```python
from build123d import *

# Parameters (mm, degrees)
SKETCH1_W           = 80
SKETCH1_H           = 20
BOSS_EXTRUDE1_DEPTH = 30
SKETCH2_W           = 80
SKETCH2_H           = 7
CUT_EXTRUDE1_DEPTH  = 22
SKETCH3_W           = 40
SKETCH3_H           = 20
BOSS_EXTRUDE2_DEPTH = 20
SKETCH4_R           = 2.25
CUT_EXTRUDE2_DEPTH  = 81.622577483
FILLET1_R           = 10
FILLET2_R           = 4


with BuildPart() as part:
    # Sketch1 → Boss-Extrude1 (new body)
    with BuildSketch(Plane(origin=(0, 0, 0), x_dir=(1, 0, 0), z_dir=(0, 1, 0))):
        with Locations((40, -10)):
            Rectangle(SKETCH1_W, SKETCH1_H)
    extrude(amount=BOSS_EXTRUDE1_DEPTH)

    # Sketch2 → Cut-Extrude1 (cut)
    with BuildSketch(Plane(origin=(0, 0, 0), x_dir=(-1, 0, 0), z_dir=(0, -1, 0))):
        with Locations((-40, -10)):
            Rectangle(SKETCH2_W, SKETCH2_H)
    extrude(amount=-CUT_EXTRUDE1_DEPTH, mode=Mode.SUBTRACT)

    # Sketch3 → Boss-Extrude2 (add)
    with BuildSketch(Plane(origin=(0, 30, 0), x_dir=(1, 0, 0), z_dir=(0, 1, 0))):
        with Locations((40, -10)):
            Rectangle(SKETCH3_W, SKETCH3_H)
    extrude(amount=BOSS_EXTRUDE2_DEPTH)

    # Sketch4 → Cut-Extrude2 (cut, through all)
    with BuildSketch(Plane.ZY.offset(-20)):
        with Locations((10, 40)):
            Circle(SKETCH4_R)
    extrude(amount=-CUT_EXTRUDE2_DEPTH, mode=Mode.SUBTRACT)

    # Fillet1
    fillet1_edges = [part.edges().sort_by_distance(p)[0] for p in [
        (40, 50, 0),
        (40, 50, 20),
    ]]
    fillet(fillet1_edges, radius=FILLET1_R - 0.0001)  # a hair under: the kernel refuses the full size

    # Fillet2
    fillet2_edges = [part.edges().sort_by_distance(p)[0] for p in [
        (40, 0, 0),
        (40, 0, 20),
    ]]
    fillet(fillet2_edges, radius=FILLET2_R)


solid = part.part
```
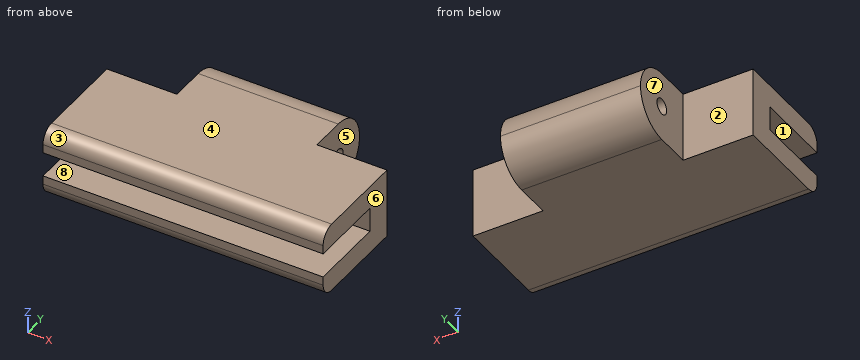
Can you work these out from the model? Positions are in its coordinate system, mm. Face numbers are marked on the shaded views. A direction names the side the tool comes from. Coordinates: 2 decimals unless noted, no trailing zeros. Loops run counter-clockwise (first coordinate to the right, second up) from the corner with the lowest first, then second, coordinate; pieces in that order, holes last. Notation, with made-up numbers: (37.5, -5) -> (62.5, -5) arc R32 ccw to (62.5, 24) -> close; hole circle Ø9 at (89.25, -40). An arc over 180 degrees is marked (long way). Answer as a JSON object with one key per item and string values.
1) Imagine slicing it at A-A (y = 17). Please give me the cut outline in (x, z).
Results:
{"outline": "(0, 0) -> (80, 0) -> (80, 6.5) -> (0, 6.5) -> close; (0, 13.5) -> (80, 13.5) -> (80, 20) -> (0, 20) -> close"}
2) Imagine slicing it at D-D (x = 17). Please give me the cut outline in (y, z), then the cut area to 3 significant figures.
Results:
{"outline": "(0, 4) arc R4 ccw to (4, 0) -> (30, 0) -> (30, 20) -> (4, 20) arc R4 ccw to (0, 16) -> (0, 13.5) -> (22, 13.5) -> (22, 6.5) -> (0, 6.5) -> close", "area": "439 mm^2"}
3) For the marked faces 4, 5, 6, 7 and 8, which set-ups out of +Z, -Z, +X, -X, +Y, -Y let a thin tool reach every point of the face, with its end or its side?
Results:
{"face 4": "+Z, +X, -X, +Y, -Y", "face 5": "+Z, -Z, +X, +Y", "face 6": "+Z, -Z, +X, +Y, -Y", "face 7": "+Z, -Z, -X, +Y", "face 8": "+X, -X, -Y"}
4) Thinking about a two-plate mould opening in Z: for the marked faces 1, 2 and 3, which applies, pulls with the +Z half, pulls with the -Z half, needs draft (parallel to the pull), parting line crosses it, or undercut?
Results:
{"face 1": "undercut", "face 2": "needs draft", "face 3": "pulls with the +Z half"}
5) For P1, Ø6, axis at x = 71.5, z = 3.5, coming from the +Y side; P2, Ø1, axis at x = 65.5, z = 11.5, coming from the -Y side; P3, Ø6, axis at y = 41.5, z = 8, coming from the -X side, each with a flat end and sliding along its axis, tell me the tip position at first contact or that it passes through.
Results:
{"P1": "stops at y = 30", "P2": "stops at y = 22", "P3": "stops at x = 20"}
6) Imagine slicing it at C-C (z = 11.25). Please give me the cut outline in (x, y).
Results:
{"outline": "(0, 22) -> (80, 22) -> (80, 30) -> (60, 30) -> (60, 38.13) -> (20, 38.13) -> (20, 30) -> (0, 30) -> close; (20, 41.87) -> (60, 41.87) -> (60, 49.92) -> (20, 49.92) -> close"}
7) If I drill on line 1 (Y direction, x = 49.5, z = 10); line 2 (Z direction, x = 23, y = 38); line 3 (X direction, y = 34, z = 7.25), over which ranges is the centre line in solid material (lowest first)?
Results:
{"line 1": "y = 22 to 37.75, 42.25 to 50", "line 2": "z = 0 to 8.97, 11.03 to 20", "line 3": "x = 20 to 60"}
